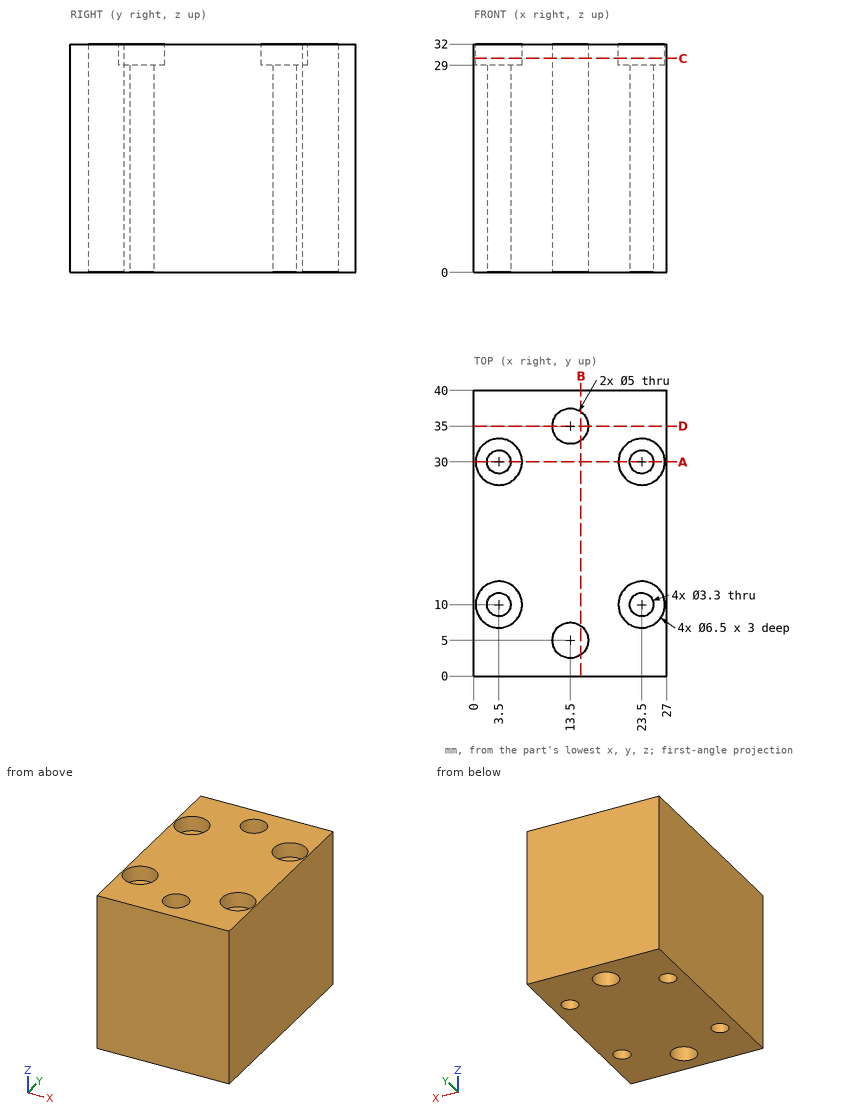
The figure shows three views and two pictorial views of one solid part (mm, origin at its lowest corner). Answer the questions. Give positions to 0.01 mm unless a question says otherwise; leave off trailing zeros. Loops run counter-clockwise (first coordinate to the right, second up) from the corner with the lowest first, then second, coordinate; pieces in that order, holes last. Notation, with made-up numbers: (17.25, 14) -> (25.25, 14) arc R20 cw to (25.25, 37) -> close; hole circle Ø6 at (47, 77.25). An arc over 180 degrees is marked (long way). Use a Markdown table: item, result. Add a question column.
1. Section A-A on y = 30 is taken. Determine the outline of the cut face in (x, z).
2. Section D-D on y = 35 is taken. Determine the outline of the cut face in (x, z).
3. Flat-ended cylindrical pins translate along their axes: pin 1 Ø5 at (x, y) = (2.5, 31.5) entering from +Z; pin 2 Ø3 at (x, y) = (13.5, 5) entering from +Z; pin 3 Ø6 at (x, y) = (3.5, 10) entering from +Z. Find the tip coordinate at first contact, or state that the pin passes through.
4. Section B-B on x = 15 is taken. Determine the outline of the cut face in (y, z), and give its area (3 significant figures).
5. Find the intervals of material crossed by probe 1 along Y at (x, z) = (3.5, 30.5); probe 2 along Y at (x, z) = (3.5, 16.75); probe 3 along Z at (x, y) = (2.75, 28.5), in increasing order.
6. Section C-C on z = 30 is taken. Determine the outline of the cut face in (x, y).
Results below:
| question | item | result |
|---|---|---|
| 1 | outline | (0, 0) -> (1.85, 0) -> (1.85, 29) -> (0.25, 29) -> (0.25, 32) -> (0, 32) -> close; (5.15, 0) -> (21.85, 0) -> (21.85, 29) -> (20.25, 29) -> (20.25, 32) -> (6.75, 32) -> (6.75, 29) -> (5.15, 29) -> close; (25.15, 0) -> (27, 0) -> (27, 32) -> (26.75, 32) -> (26.75, 29) -> (25.15, 29) -> close |
| 2 | outline | (0, 0) -> (11, 0) -> (11, 32) -> (0, 32) -> close; (16, 0) -> (27, 0) -> (27, 32) -> (16, 32) -> close |
| 3 | pin 1 | stops at z = 32 |
| 3 | pin 2 | passes through |
| 3 | pin 3 | stops at z = 29 |
| 4 | outline | (0, 0) -> (3, 0) -> (3, 32) -> (0, 32) -> close; (7, 0) -> (33, 0) -> (33, 32) -> (7, 32) -> close; (37, 0) -> (40, 0) -> (40, 32) -> (37, 32) -> close |
| 4 | area | 1,020 mm^2 |
| 5 | probe 1 | y = 0 to 6.75, 13.25 to 26.75, 33.25 to 40 |
| 5 | probe 2 | y = 0 to 8.35, 11.65 to 28.35, 31.65 to 40 |
| 5 | probe 3 | z = 0 to 29 |
| 6 | outline | (0, 0) -> (27, 0) -> (27, 40) -> (0, 40) -> close; hole circle Ø6.5 at (3.5, 10); hole circle Ø6.5 at (3.5, 30); hole circle Ø5 at (13.5, 5); hole circle Ø5 at (13.5, 35); hole circle Ø6.5 at (23.5, 10); hole circle Ø6.5 at (23.5, 30) |
